Geometry check sheet. Reference: the model listing, model coordinates, mm. Face numbers are marked on the shaded views. Round coordinates to 2 decimals unless told otherwise and drop trailing zeros. Write each loop counter-clockwise with the first axis right and the second up, starting at its lowest first coordinate (ties: lowest second). Pieces come first, ordered by that corner, then holes.
Item 1: Cross-section at D-D (z = 3.15). Enter the section's corners in (x, y).
Item 2: Cross-section at C-C (y = -4). Enter the section's corners in (x, z).
Item 3: Depth check by flat-ended pin: P1, Ø1, axis at y = 1.5, z = 2.5, coming from the +X side; P2, Ø1, axis at x = -5, z = 2.5, coming from the -Y side; P3, Ø2, axis at y = -7, z = 3.5, coming from the +X side. Enter the tip coordinate at first touch or a pass-through.
Item 4: Draft check along X on the marked faces 1, 2 and 3. Enter one of: pulls with the +X half, pulls with the -X half, needs draft (parallel to the pull), parting line crosses it, or undercut.
Item 5: Cross-section at A-A (y = 9). Enter the section's corners in (x, z).
Item 6: Scan lines: probe 1 along Y at (x, z) = (0, 3.9); probe 2 along Y at (x, z) = (-8.5, 1.75); probe 3 along X at (y, z) = (5, 0.2). Record each from-to range of solid material in increasing order.
Item 7: Cross-section at B-B (x = 0). Enter the section's corners in (y, z).
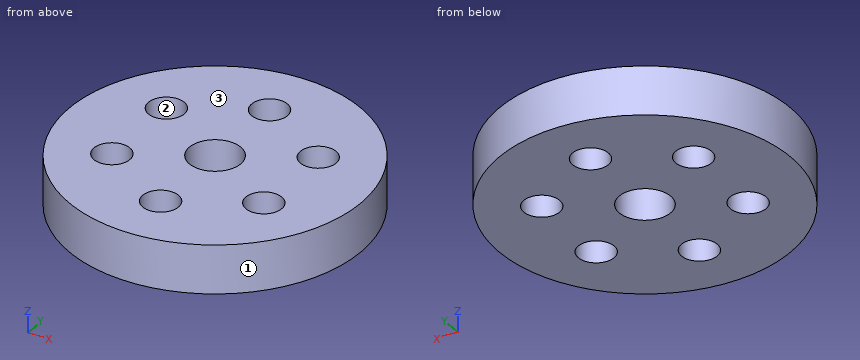
from build123d import *

# Parameters (mm, degrees)
SKETCH_1_R               = 15
EXTRUDE_1_DEPTH          = 5
HOLE_WIZARD_M5_1_D       = 5.3
HOLE_WIZARD_M3_5_1_D     = 3.7
PATTERN_CIRCULAR_1_COUNT = 6


with BuildPart() as part:
    # ｽｹｯﾁ1 → ﾎﾞｽ - 押し出し1 (new body)
    with BuildSketch(Plane.XY):
        Circle(SKETCH_1_R)
    extrude(amount=EXTRUDE_1_DEPTH)

    # M5 すきま穴1 (through all)
    with Locations(Plane(origin=(0, 0, 0), x_dir=(-1, 0, 0), z_dir=(0, 0, -1))):
        with Locations((0, 0)):
            Hole(HOLE_WIZARD_M5_1_D / 2)

    # M3.5 すきま穴1 (through all)
    with Locations(Plane(origin=(0, 9, 0), x_dir=(-1, 0, 0), z_dir=(0, 0, -1))):
        with Locations((0, 0)):
            hole_wizard_m3_5_1 = Hole(HOLE_WIZARD_M3_5_1_D / 2)

    # 円形ﾊﾟﾀｰﾝ1: M3.5 すきま穴1 ×6 about axis
    pattern_circular_1_axis = Axis((0, 0, 0), (0, 0, 1))
    for i in range(1, PATTERN_CIRCULAR_1_COUNT):
        add(hole_wizard_m3_5_1.rotate(pattern_circular_1_axis, i * 360 / PATTERN_CIRCULAR_1_COUNT), mode=Mode.SUBTRACT)


solid = part.part
Resolved:
1. outline: circle Ø30 at (0, 0); hole circle Ø3.7 at (-7.79, -4.5); hole circle Ø3.7 at (-7.79, 4.5); hole circle Ø5.3 at (0, 0); hole circle Ø3.7 at (0, -9); hole circle Ø3.7 at (0, 9); hole circle Ø3.7 at (7.79, -4.5); hole circle Ø3.7 at (7.79, 4.5)
2. outline: (-14.46, 0) - (-9.58, 0) - (-9.58, 5) - (-14.46, 5) - close; (-6.01, 0) - (6.01, 0) - (6.01, 5) - (-6.01, 5) - close; (9.58, 0) - (14.46, 0) - (14.46, 5) - (9.58, 5) - close
3. P1: stops at x = 14.97
3. P2: stops at y = -14.31
3. P3: stops at x = 13.75
4. face 1: parting line crosses it
4. face 2: undercut
4. face 3: needs draft
5. outline: (-12, 0) - (-1.85, 0) - (-1.85, 5) - (-12, 5) - close; (1.85, 0) - (12, 0) - (12, 5) - (1.85, 5) - close
6. probe 1: y = -15 to -10.85, -7.15 to -2.65, 2.65 to 7.15, 10.85 to 15
6. probe 2: y = -12.36 to -6.21, -2.79 to 2.79, 6.21 to 12.36
6. probe 3: x = -14.14 to -9.58, -6.01 to 6.01, 9.58 to 14.14
7. outline: (-15, 0) - (-10.85, 0) - (-10.85, 5) - (-15, 5) - close; (-7.15, 0) - (-2.65, 0) - (-2.65, 5) - (-7.15, 5) - close; (2.65, 0) - (7.15, 0) - (7.15, 5) - (2.65, 5) - close; (10.85, 0) - (15, 0) - (15, 5) - (10.85, 5) - close
